The figure shows three views and two pictorial views of one solid part (mm, origin at its lowest corner). Answer the questions. A direction names the side the tool comes from. Round coordinates to 2 decimals unless told otherwise and drop trailing zeros. Order: outer loops, then holes, each group sorted by start corner. A loop starts at its lowest first (then second) coordinate and runs counter-clockwise, first axis right, second up. Notation, with made-up numbers: (-40, 81.5) - (9, 81.5) arc R24 ccw to (9, 117.5) - close; hole circle Ø11 at (15, 75). An arc over 180 degrees is marked (long way). Use CSV: the item, a comma, the result in double quotes.
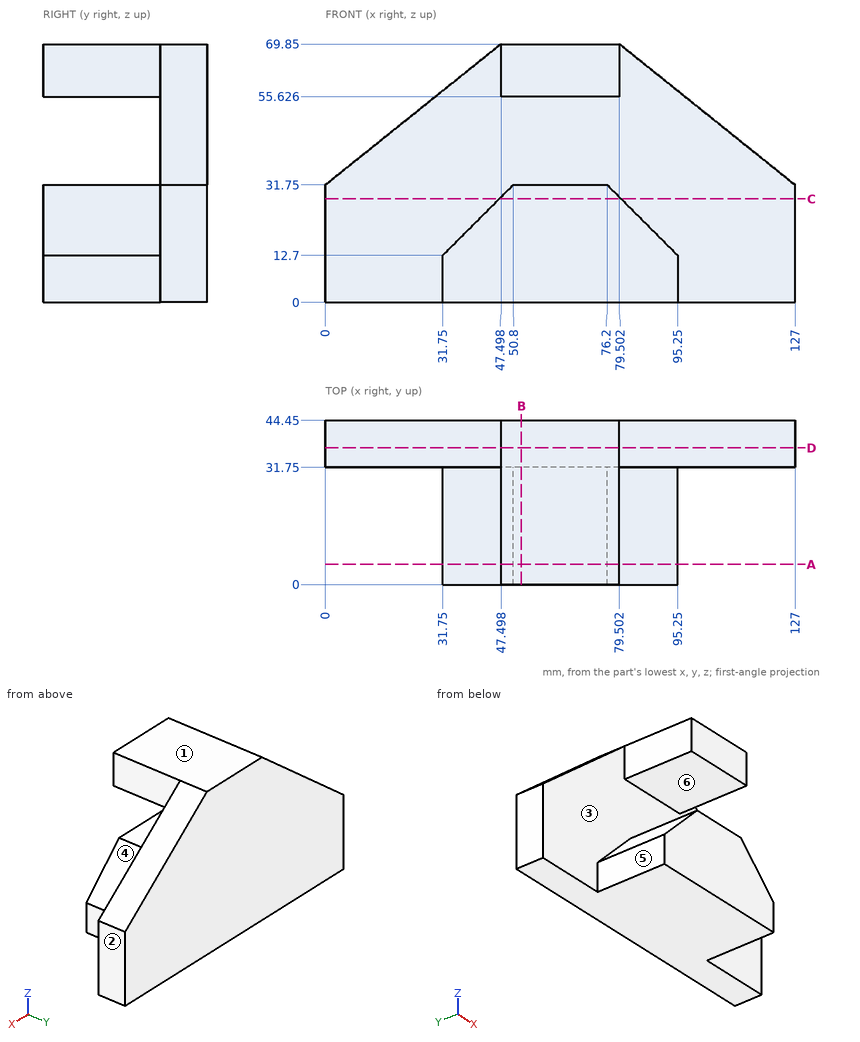
(1) Find section D-D (y = 37). Determine the outline of the cut face in (x, z), and give its area (3 significant figures).
Findings below:
outline,"(0, 0) - (127, 0) - (127, 31.75) - (79.5, 69.85) - (47.5, 69.85) - (0, 31.75) - close"
area,"7,060 mm²"
(2) For the marked faces 4, 5 and 6, determine the directions among +Z, -Z, +X, -X, +Y, -Y from which every point of the face is accessible in a straight line to the end or side of a thin tool.
Findings below:
face 4,"+X, -Y"
face 5,"+Z, -Z, -X, -Y"
face 6,"+X, -X, -Y"
(3) Find section A-A (y = 5.5). Determine the outline of the cut face in (x, z), and give its area (3 significant figures).
Findings below:
outline,"(31.75, 0) - (95.25, 0) - (95.25, 12.7) - (76.2, 31.75) - (50.8, 31.75) - (31.75, 12.7) - close; (47.5, 55.63) - (79.5, 55.63) - (79.5, 69.85) - (47.5, 69.85) - close"
area,"2,110 mm²"
(4) Each of these flat-tipped pins is pushed along its axis until it touches: pin 1 (14 mm diameter, centred on y = 19, z = 7.5, fed in from +X); pin 2 (1.5 mm diameter, centred on y = 13.5, z = 16, fed in from +X); pin 3 (6 mm diameter, centred on x = 101, z = 58, fed in from -Y); pin 4 (1 mm diameter, centred on y = 33.5, z = 51.5, fed in from -X). Where does it stop, or does it pass through?
Findings below:
pin 1,"stops at x = 95.25"
pin 2,"stops at x = 92.7"
pin 3,"passes through"
pin 4,"stops at x = 24"
(5) Find section B-B (x = 53). Determine the outline of the cut face in (y, z).
Findings below:
outline,"(0, 0) - (44.45, 0) - (44.45, 69.85) - (0, 69.85) - (0, 55.63) - (31.75, 55.63) - (31.75, 31.75) - (0, 31.75) - close"
(6) Find section C-C (z = 28). Determine the outline of the cut face in (x, y).
Findings below:
outline,"(0, 31.75) - (47.05, 31.75) - (47.05, 0) - (79.95, 0) - (79.95, 31.75) - (127, 31.75) - (127, 44.45) - (0, 44.45) - close"
(7) Find the intervals of material crossed by L1, parallel to Z at x = 76, y = 17; L2, parallel to X at y = 27, z = 11; L3, parallel to Y at x = 77.5, z = 53, in increasing order. Write a range as from..to.
Findings below:
L1,"z = 0..31.75, 55.63..69.85"
L2,"x = 31.75..95.25"
L3,"y = 31.75..44.45"
(8) The mould has two halves that part along Z. Classify the marked faces 1, 2 and 3: released by +Z, released by -Z, zero draft, split by the parting line, or undercut.
Findings below:
face 1,"released by +Z"
face 2,"zero draft"
face 3,"undercut"
